Geometry: see drawing. Coordinates: mm, zero at the bounding-box minimum. A direction names the side the tool comes from. Give positions to 0.01 mm unless a question says otherwise; leave off trailing zeros. Write each loop counter-clockwise with the first axis right and the second up, starting at its lowest first coordinate (ties: lowest second). Pieces come first, ordered by that corner, then holes.
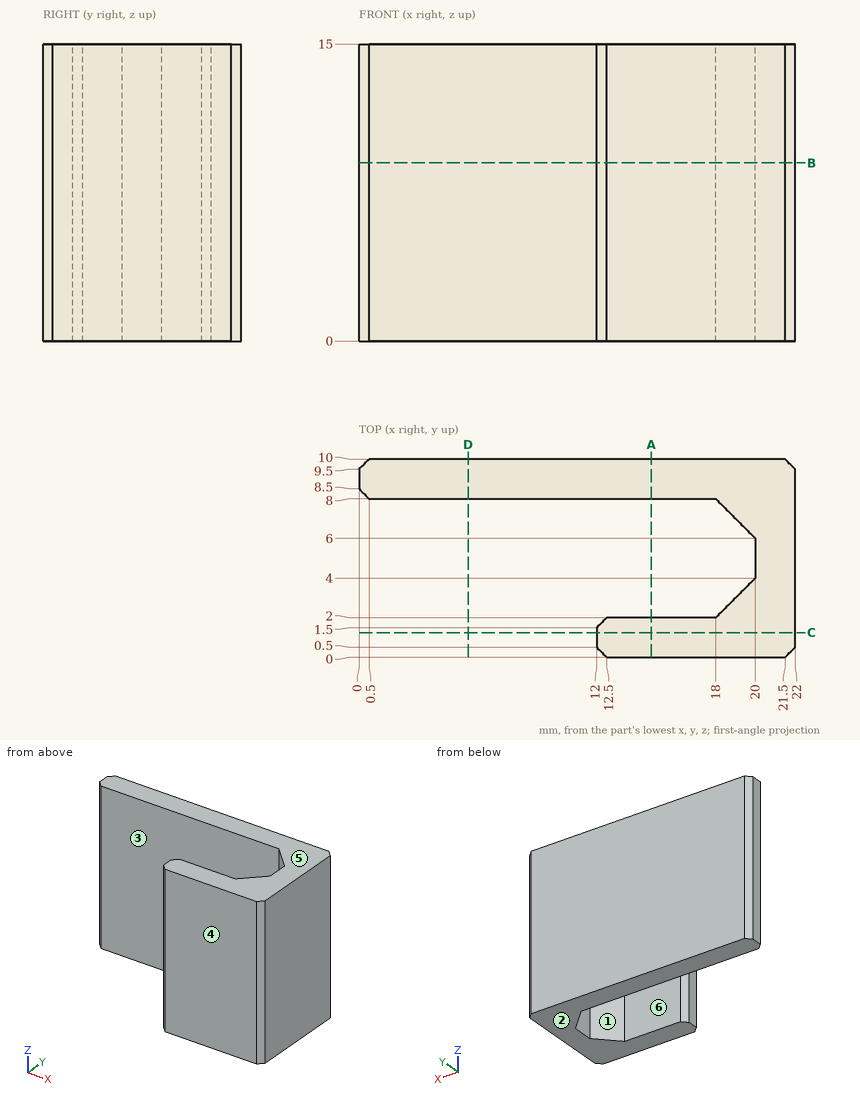
1. Section query B-B (z = 9). Return loops of the section in (x, y), plus the area to 4 significant figures.
2. Pull-direction query (Y, two-part tool) for the marked faces 3, 4, 5 and 6; classes: pulls with the +Y half, pulls with the -Y half, needs draft (parallel to the pull), parting line crosses it, or undercut.
3. Section query A-A (x = 14.75). Return loops of the section in (y, z).
4. Section query D-D (x = 5.5). Return loops of the section in (y, z), plus the area to 3 significant figures.
5. Pin query (flat end, axial travel): P1, Ø1.1, axis at y = 1, z = 7.5, coming from the -X side. Return the tip coordinate at first contact, or that it passes through.
6. Line query: probe 1 along Y at (x, z) = (13.25, 11.5); probe 2 along X at (y, z) = (5, 11.25); probe 3 along Y at (x, z) = (3, 3.75). Output: solid intervals per line, ascending.
7. Access query for the marked faces 1 and 2. Directions: +Z, -Z, +X, -X, +Y, -Y. A direction counts if a zero-diameter tool reaches every point of the face in a straight line with its end or side. Return the directions, or none.
8. Section query C-C (y = 1.25). Return loops of the section in (x, z).
The answers:
1. outline: (0, 8.5) - (0.5, 8) - (18, 8) - (20, 6) - (20, 4) - (18, 2) - (12.5, 2) - (12, 1.5) - (12, 0.5) - (12.5, 0) - (21.5, 0) - (22, 0.5) - (22, 9.5) - (21.5, 10) - (0.5, 10) - (0, 9.5) - close
1. area: 79.25 mm2
2. face 3: undercut
2. face 4: pulls with the -Y half
2. face 5: needs draft
2. face 6: undercut
3. outline: (0, 0) - (2, 0) - (2, 15) - (0, 15) - close; (8, 0) - (10, 0) - (10, 15) - (8, 15) - close
4. outline: (8, 0) - (10, 0) - (10, 15) - (8, 15) - close
4. area: 30.0 mm2
5. P1: stops at x = 12
6. probe 1: y = 0 to 2, 8 to 10
6. probe 2: x = 20 to 22
6. probe 3: y = 8 to 10
7. face 1: +Z, -Z, -X
7. face 2: -Z, +X, -X, +Y, -Y
8. outline: (12, 0) - (22, 0) - (22, 15) - (12, 15) - close
